Could you check a few things on this model? Use its own coordinates, in mm. Face numbers are marked on the shaded views. A direction names the side the tool comes from. Round coordinates to 2 decimals unless told otherwise and drop trailing zeros. Loops run counter-clockwise (first coordinate to the right, second up) from the corner with the lowest first, then second, coordinate; pieces in that order, holes last. Notation, with made-up numbers: (84.25, -1) -> (132.25, -1) arc R15 cw to (132.25, 23) -> close; hole circle Ø4 at (72.25, 44). An arc over 180 degrees is marked (long way). One line per item, written item: value.
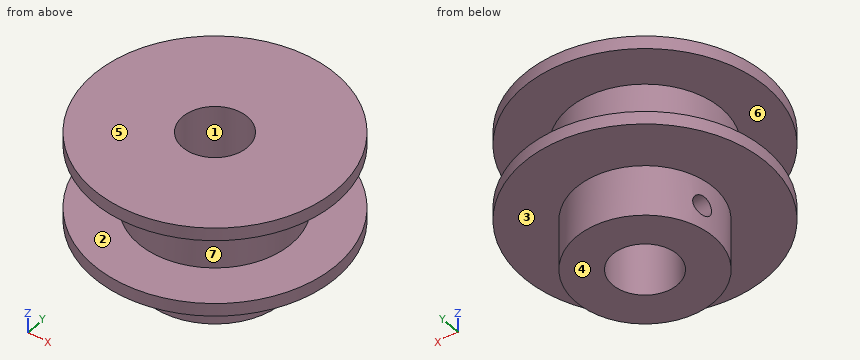
Autodesk Inventor part; units mm, degrees
ref_plane "YZ Plane" through (0, 0, 0) normal (1, 0, 0) x (0, 1, 0)
ref_plane "XZ Plane" through (0, 0, 0) normal (0, 1, 0) x (-1, 0, 0)
ref_plane "XY Plane" through (0, 0, 0) normal (0, 0, 1) x (1, 0, 0)
sketch "Sketch1" plane through (0, 0, 0) normal (1, 0, 0) x (0, 1, 0)
  line L0 (0, 17.5) -> (11, 17.5)
  line L1 (11, 17.5) -> (11, 15.9)
  line L2 (11, 15.9) -> (5.445, 15.9)
  line L3 (5.445, 15.9) -> (5.445, 7.9)
  line L4 (5.445, 7.9) -> (11, 7.9)
  line L5 (11, 7.9) -> (11, 6.3)
  line L6 (11, 6.3) -> (4.5, 6.3)
  line L7 (4.5, 6.3) -> (4.5, 0)
  line L8 (4.5, 0) -> (0, 0)
  line L9 (0, 0) -> (0, 17.5)
  line L10 (-4, 10.0812) -> (-4, 1.7277) construction
  dimension "d0" = 30
  dimension "d1" = 17.5
  dimension "d2" = 8
  dimension "d3" = 11.2
  dimension "d4" = 8
  dimension "d5" = 17
  dimension "d6" = 18.89
revolve "Revolution1" add sketch "Sketch1" angle 360 about axis through (0, -4, 10.0812) along (0, 0, -1)
sketch "Sketch2" plane through (0, 0, 0) normal (1, 0, 0) x (0, 1, 0)
  line L0 (-12.5, 6.3) -> (-12.5, 0) construction
  line L1 (4.5, 6.3) -> (4.5, 0) construction
  line L2 (-12.5, 0) -> (4.5, 0) construction
  line L3 (-11.6, 0) -> (6.6, 0) construction
  point P0 (0, 0)
  point P1 (-2.5, 3)
  point P2 (-2.5, 3)
  dimension "d8" = 3
hole "Hole1" at (0, -2.5, 3) direction (-1, 0, 0) diameter 2.459 end through all
(1) If we section it at C-C, the plane x = -5.5: Please give me the cut outline in (y, z).
Recorded:
outline: (-17.96, 6.3) -> (-10.48, 6.3) -> (-10.48, 0) -> (2.48, 0) -> (2.48, 6.3) -> (9.96, 6.3) -> (9.96, 7.9) -> (3.68, 7.9) -> (3.68, 15.9) -> (9.96, 15.9) -> (9.96, 17.5) -> (-17.96, 17.5) -> (-17.96, 15.9) -> (-11.68, 15.9) -> (-11.68, 7.9) -> (-17.96, 7.9) -> close; hole circle Ø2.46 at (-2.5, 3)
(2) Thinking about a two-plate mould opening in Z: for the marked faces 4, 5, 6 and 7, which applies, released by +Z, released by -Z, zero draft, split by the parting line, or undercut?
Recorded:
face 4: released by -Z
face 5: released by +Z
face 6: undercut
face 7: undercut
(3) If I drill on L1, parallel to Z at x = -13, y = -9.75; L2, parallel to X at y = -4, z = 13 (3 decimals); L3, parallel to Z at x = -6.65, y = -2.5, over which ranges is the centre line in solid material (lowest first)?
Recorded:
L1: 6.3 to 7.9, 15.9 to 17.5
L2: -9.445 to -4, 4 to 9.445
L3: 0 to 1.77, 4.23 to 17.5
(4) If we section it at A-A, the plane x = -12: Please give me the cut outline in (y, z).
Recorded:
outline: (-13, 6.3) -> (5, 6.3) -> (5, 7.9) -> (-13, 7.9) -> close; (-13, 15.9) -> (5, 15.9) -> (5, 17.5) -> (-13, 17.5) -> close
(5) I'm going to push flat-ended pins straight in: pin 1 Ø1 at (y, z) = (4, 10) entering from +X; pin 2 Ø1.5 at (y, z) = (-8.5, 14) entering from -X; pin 3 Ø5 at (x, y) = (11, -13) entering from -Z. Where does each tip first touch, or does it pass through?
Recorded:
pin 1: x = 5.74
pin 2: x = -8.67
pin 3: z = 6.3
(6) For the marked faces 1, 2 and 3, which set-ups out of +Z, -Z, +X, -X, +Y, -Y let a thin tool reach every point of the face, with its end or its side?
Recorded:
face 1: +Z, -Z
face 2: none
face 3: -Z
(7) If we section it at B-B, the plane y = -2.5: Please give me the cut outline in (x, z), then the cut area to 3 significant figures.
Recorded:
outline: (-14.92, 6.3) -> (-8.37, 6.3) -> (-8.37, 4.23) -> (-3.71, 4.23) -> (-3.71, 17.5) -> (-14.92, 17.5) -> (-14.92, 15.9) -> (-9.33, 15.9) -> (-9.33, 7.9) -> (-14.92, 7.9) -> close; (-8.37, 0) -> (-3.71, 0) -> (-3.71, 1.77) -> (-8.37, 1.77) -> close; (3.71, 0) -> (8.37, 0) -> (8.37, 6.3) -> (14.92, 6.3) -> (14.92, 7.9) -> (9.33, 7.9) -> (9.33, 15.9) -> (14.92, 15.9) -> (14.92, 17.5) -> (3.71, 17.5) -> close
area: 209 mm²
(8) If we section it at D-D, the plane z = 5.5: Please give me the cut outline in (x, y).
Recorded:
outline: circle Ø17 at (0, -4); hole circle Ø8 at (0, -4)
